Answer from the drawing. Dimensions are ordinates in mm from the lowest x, y and z of the part. Coordinates: 2 decimals unless noted, no trailing zeros. Write each loop counter-clockwise with the first axis right and the second up, starting at its lowest first coordinate (ties: lowest second). Pieces come first, ordered by that corner, then holes. Notation, with made-up numbers: (39.25, 48.5) -> (72.25, 48.5) arc R18 cw to (72.25, 79.5) -> close; hole circle Ø10 at (31, 62). An arc over 180 degrees is marked (long way). One line per item, written item: value. Start each with the question number.
1. Find section B-B, the plane x = 251. Write down the section's boundary in (y, z).
2. Find section C-C, the plane z = 10.25. Write down the section's boundary in (x, y).
3. Find section A-A, the plane y = 2.3. Write down the section's boundary in (x, z).
4. Consider line 1 along X through (y, z) = (2.1, 16); line 2 along X through (y, z) = (2.6, 27.25); line 3 along X through (y, z) = (0.8, 15.25). Determine where each line is inside the solid, lowest interval first.
5. Given P1, Ø1, axis at y = 1, z = 20, coming from the -X side, flat-ended and moving along its own axis, determine where the tip first touches the part or whether it passes through.
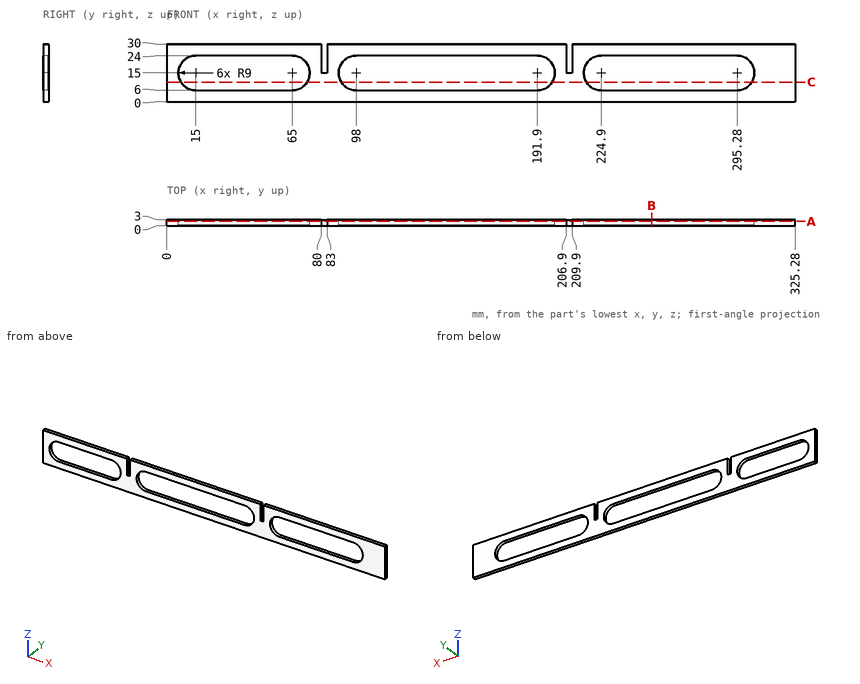
Answer block:
1. outline: (0, 0) -> (3, 0) -> (3, 6) -> (0, 6) -> close; (0, 24) -> (3, 24) -> (3, 30) -> (0, 30) -> close
2. outline: (0, 0) -> (7.36, 0) -> (7.36, 3) -> (0, 3) -> close; (72.64, 0) -> (90.36, 0) -> (90.36, 3) -> (72.64, 3) -> close; (199.54, 0) -> (217.26, 0) -> (217.26, 3) -> (199.54, 3) -> close; (302.92, 0) -> (325.28, 0) -> (325.28, 3) -> (302.92, 3) -> close
3. outline: (0, 0) -> (325.28, 0) -> (325.28, 30) -> (209.9, 30) -> (209.9, 15) -> (206.9, 15) -> (206.9, 30) -> (83, 30) -> (83, 15) -> (80, 15) -> (80, 30) -> (0, 30) -> close; hole (15, 6) -> (65, 6) arc R9 ccw to (65, 24) -> (15, 24) arc R9 ccw to start; hole (98, 6) -> (191.9, 6) arc R9 ccw to (191.9, 24) -> (98, 24) arc R9 ccw to start; hole (224.9, 6) -> (295.28, 6) arc R9 ccw to (295.28, 24) -> (224.9, 24) arc R9 ccw to start
4. line 1: x = 0 to 6.06, 73.94 to 80, 83 to 89.06, 200.84 to 206.9, 209.9 to 215.96, 304.22 to 325.28
4. line 2: x = 0 to 80, 83 to 206.9, 209.9 to 325.28
4. line 3: x = 0 to 6, 74 to 80, 83 to 89, 200.9 to 206.9, 209.9 to 215.9, 304.28 to 325.28
5. P1: stops at x = 0
